Answer from the drawing. Dimensions are ordinates in mm from the lowest x, y and z of the part. A direction names the side the tool comes from. Round coordinates to 2 decimals unless told otherwise and drop trailing zeros. Write each loop counter-clockwise with the first axis right and the second up, starting at its lowest first coordinate (ties: lowest second). Pieces come first, ordered by that corner, then holes. Notation, with made-up numbers: (-29.5, 21) - (25.5, 21) arc R15 ccw to (25.5, 46) - close; hole circle Ø3 at (0.25, 54). An arc over 180 degrees is marked (long way). One line per item, written item: value. Start each with the question number.
(1) For the marked faces 1, 2, 3, 4 and 5, determine the directions among +Z, -Z, +X, -X, +Y, -Y from which every point of the face is accessible in a straight line to the end or side of a thin tool.
(2) A cutting plane is placed at B-B, the plane y = 15.5. Determine the outline of the cut face in (x, z).
(3) Find the intervals of material crossed by L1, parallel to X at y = 18, z = 19.25; L2, parallel to Z at x = 39.5, y = 18; L3, parallel to X at y = 2.5, z = 2.5, in increasing order.
(4) A cutting plane is placed at D-D, the plane z = 4.5. Determine the outline of the cut face in (x, y), plus the area to 3 significant figures.
(5) A cutting plane is placed at A-A, the plane z = 14.75. Determine the outline of the cut face in (x, y), plus the area to 3 significant figures.
(6) A cutting plane is placed at C-C, the plane x = 15.5. Determine the outline of the cut face in (y, z).
(7) Flat-ended cylindrical pins translate along their axes: pin 1 Ø4 at (x, y) = (55.5, 11.5) entering from +Z; pin 2 Ø1 at (y, z) = (12, 3.5) entering from +X; pin 3 Ø4 at (y, z) = (7.5, 18) entering from -X. Find the tip coordinate at first contact, or state that the pin passes through.
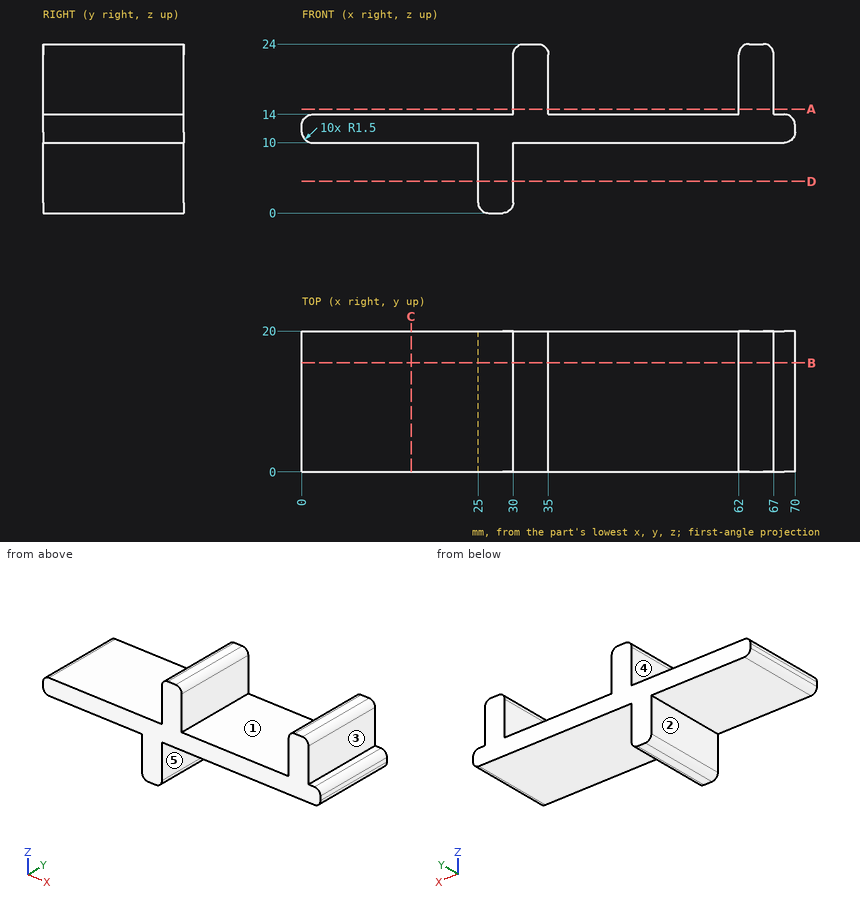
Here are the results:
1. face 1: +Z, +Y, -Y
1. face 2: -Z, -X, +Y, -Y
1. face 3: +Z, +X, +Y, -Y
1. face 4: +Z, -X, +Y, -Y
1. face 5: -Z, +X, +Y, -Y
2. outline: (0, 11.5) arc R1.5 ccw to (1.5, 10) - (25, 10) - (25, 1.5) arc R1.5 ccw to (26.5, 0) - (28.5, 0) arc R1.5 ccw to (30, 1.5) - (30, 10) - (68.5, 10) arc R1.5 ccw to (70, 11.5) - (70, 12.5) arc R1.5 ccw to (68.5, 14) - (67, 14) - (67, 22.5) arc R1.5 ccw to (65.5, 24) - (63.5, 24) arc R1.5 ccw to (62, 22.5) - (62, 14) - (35, 14) - (35, 22.5) arc R1.5 ccw to (33.5, 24) - (31.5, 24) arc R1.5 ccw to (30, 22.5) - (30, 14) - (1.5, 14) arc R1.5 ccw to (0, 12.5) - close
3. L1: 30 to 35, 62 to 67
3. L2: 10 to 14
3. L3: 25 to 30
4. outline: (25, 0) - (30, 0) - (30, 20) - (25, 20) - close
4. area: 100 mm²
5. outline: (30, 0) - (35, 0) - (35, 20) - (30, 20) - close; (62, 0) - (67, 0) - (67, 20) - (62, 20) - close
5. area: 200 mm²
6. outline: (0, 10) - (20, 10) - (20, 14) - (0, 14) - close
7. pin 1: z = 14
7. pin 2: x = 30
7. pin 3: x = 30
